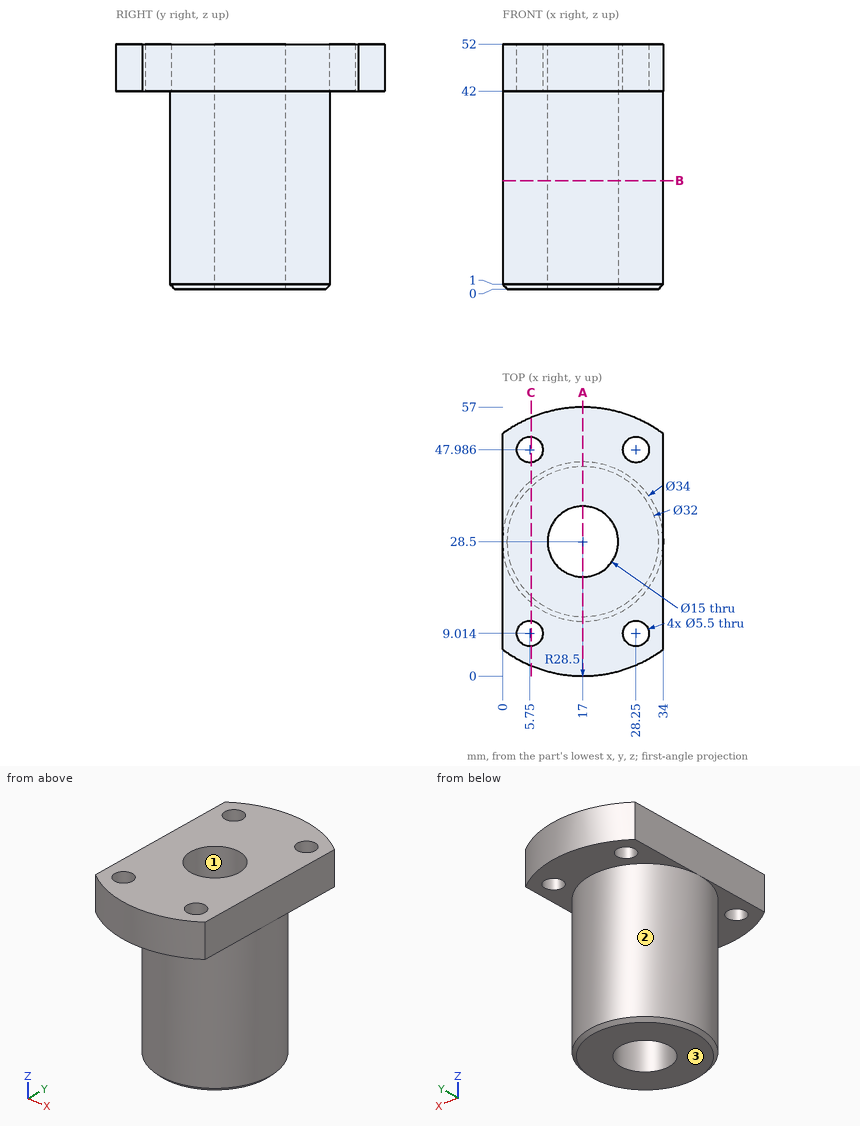
For this review, use the dimensioned drawing (mm, ordinates from the lowest corner) and the shaded views. Round coordinates to 2 decimals unless told otherwise and drop trailing zeros. Write each loop counter-clockwise with the first axis right and the second up, starting at its lowest first coordinate (ties: lowest second). Pieces come first, ordered by that corner, then holes. Notation, with made-up numbers: (-1.5, 13) -> (36.5, 13) arc R18 cw to (36.5, 22) -> close; hole circle Ø9 at (7.5, -22.5). An arc over 180 degrees is marked (long way). Answer in a Markdown table with one row per item.
Q1. To check wall thickness, follow L1, parallel to X at y = 28, z = 25; L2, parallel to Y at x = 5, z = 46; L3, parallel to Y at x = 5.75, z = 50 (1 decimal). State the ranges of each line that lie inside material, in increasing order. Write a range as [from, to].
The answers:
| item | result |
|---|---|
| L1 | [0.01, 9.52], [24.48, 33.99] |
| L2 | [2.65, 6.37], [11.66, 45.34], [50.63, 54.35] |
| L3 | [2.3, 6.3], [11.8, 45.2], [50.7, 54.7] |
Q2. Draft analysis for pull direction X (two halves, no side actions). For the marked faces 1, 2 and 3, state which applies: +X half, -X half, draft (parallel to the pull), parting line (faces both ways), or undercut.
The answers:
| item | result |
|---|---|
| face 1 | undercut |
| face 2 | parting line |
| face 3 | draft |
Q3. Clearance check with flat-ended pins moving along their axes: pin 1 Ø3.5 at (x, y) = (28.25, 9.01) entering from +Z; pin 2 Ø1 at (x, z) = (14.5, 46.5) entering from -Y; pin 3 Ø12 at (x, z) = (18, 12) entering from +Y; pin 4 Ø7 at (x, y) = (5.75, 47.99) entering from -Z. State where each tip first meets the part, or that it passes through.
The answers:
| item | result |
|---|---|
| pin 1 | through |
| pin 2 | y = 0.07 |
| pin 3 | y = 45.5 |
| pin 4 | z = 42 |
Q4. Take a section at C-C, the plane x = 6. Count the separate pieces of the cut face and the enclosed holes in it, then the cut area to 3 significant figures.
The answers:
| item | result |
|---|---|
| separate pieces | 3 |
| enclosed holes | 0 |
| area | 1,500 mm² |
Q5. Take a section at B-B, the plane z = 23. State the section outline as (x, y) points.
The answers:
| item | result |
|---|---|
| outline | circle Ø34 at (17, 28.5); hole circle Ø15 at (17, 28.5) |
Q6. Take a section at A-A, the plane x = 17. State the section outline as (y, z) points.
The answers:
| item | result |
|---|---|
| outline | (0, 42) -> (11.5, 42) -> (11.5, 1) -> (12.5, 0) -> (21, 0) -> (21, 52) -> (0, 52) -> close; (36, 0) -> (44.5, 0) -> (45.5, 1) -> (45.5, 42) -> (57, 42) -> (57, 52) -> (36, 52) -> close |
